CAD build for the part. Positions are in the model's coordinates, mm. A direction names the side the tool comes from. Coordinates: 2 decimals unless noted, no trailing zeros. Write each loop counter-clockwise with the first axis right and the second up, starting at its lowest first coordinate (ties: lowest second). Pieces come first, ordered by that corner, then holes. Notation, with made-up numbers: (45.25, 89.25) - (68.25, 89.25) arc R23 cw to (68.25, 117.25) - close; hole circle Ø7 at (-21.75, 38.25). An arc over 180 degrees is marked (long way). Answer in a Markdown table with one row per item. Add a question column.
Q1. Band-saw the part on D-D (x = 6.5). List the corners of the cut face in (y, z).
Q2. Drill centre lines: line 1 along Y through (x, z) = (0, 4.5); line 2 along Y through (x, z) = (0, -2.4); line 3 along Z through (x, y) = (2, 1.5). Where is each one in solid material? Low to high. Write a range as from..to.
Q3. Pin check, flat tips, straight feed: pin 1 (1.5 mm diameter, centred on y = 3.5, z = 2, fed in from -X); pin 2 (5 mm diameter, centred on x = -1, y = 5, fed in from +Z); pin 3 (1 mm diameter, centred on x = -1.5, z = 2.5, fed in from +Y). Stop position of each tip, or through.
Q4. Two-plate mould, pull along X, no slides. Class faces 1 (the flat face through (0, 0, -1)), 2 (the flat face through (0, 0, 0)), 3 (the flat face through (5.2, 0.2, -3)), 4 (the cylindrical face through (-11.99, 0.53, 2.83)): +X half, -X half, draft (parallel to the pull), parting line (faces both ways), or undercut.
Q5. 3-axis set-ups, long thin cutter, end or side, ignore diameter. For faces 5 (the cylindrical face through (-1.172, 8.923, 4.19)), 6 (the flat face through (2, 9, 8.5)), 7 (the cylindrical face through (1.08, -4.88, -2.01)): which of +Z, -Z, +X, -X, +Y, -Y reach the whole face in a straight line?
Q6. Band-saw the part on A-A (x = 0). List the corners of the cut face in (y, z).
Q7. Band-saw the part on C-C (z = 3.75). List the corners of the cut face in (x, y), and give its area (3 significant figures).
```python
from build123d import *

# Parameters (mm, degrees)
SKETCH1_R           = 12
SKETCH1_R_2         = 9
BOSS_EXTRUDE1_DEPTH = 8.5
SKETCH1_2_R         = 12
BOSS_EXTRUDE2_DEPTH = 3
SKETCH2_R           = 5
CUT_EXTRUDE1_DEPTH  = 2


with BuildPart() as part:
    # Sketch1 → Boss-Extrude1 (new body)
    with BuildSketch(Plane.XY):
        Circle(SKETCH1_R)
        Circle(SKETCH1_R_2, mode=Mode.SUBTRACT)
    extrude(amount=BOSS_EXTRUDE1_DEPTH)

    # Sketch1_2 → Boss-Extrude2 (add)
    with BuildSketch(Plane.XY):
        Circle(SKETCH1_2_R)
    extrude(amount=-BOSS_EXTRUDE2_DEPTH)

    # Sketch2 → Cut-Extrude1 (cut)
    with BuildSketch(Plane(origin=(0, 0, -3), x_dir=(-1, 0, 0), z_dir=(0, 0, -1))):
        Circle(SKETCH2_R)
    extrude(amount=-CUT_EXTRUDE1_DEPTH, mode=Mode.SUBTRACT)


solid = part.part
```
Checked values:
| question | item | result |
|---|---|---|
| 1 | outline | (-10.09, -3) - (10.09, -3) - (10.09, 8.5) - (6.22, 8.5) - (6.22, 0) - (-6.22, 0) - (-6.22, 8.5) - (-10.09, 8.5) - close |
| 2 | line 1 | y = -12..-9, 9..12 |
| 2 | line 2 | y = -12..-5, 5..12 |
| 2 | line 3 | z = -1..0 |
| 3 | pin 1 | stops at x = -11.68 |
| 3 | pin 2 | stops at z = 0 |
| 3 | pin 3 | stops at y = 11.96 |
| 4 | face 1 | undercut |
| 4 | face 2 | undercut |
| 4 | face 3 | draft |
| 4 | face 4 | parting line |
| 5 | face 5 | +Z |
| 5 | face 6 | +Z, +X, -X, +Y, -Y |
| 5 | face 7 | -Z |
| 6 | outline | (-12, -3) - (-5, -3) - (-5, -1) - (5, -1) - (5, -3) - (12, -3) - (12, 8.5) - (9, 8.5) - (9, 0) - (-9, 0) - (-9, 8.5) - (-12, 8.5) - close |
| 7 | outline | circle Ø24 at (0, 0); hole circle Ø18 at (0, 0) |
| 7 | area | 198 mm² |
